Work out the finished part from the listing and answer in its coordinate system (mm). Face numbers are marked on the shaded views. A direction names the side the tool comes from. Round coordinates to 2 decimals unless told otherwise and drop trailing zeros. Order: outer loops, then holes, each group sorted by start corner. A loop starts at its lowest first (then second) coordinate and runs counter-clockwise, first axis right, second up. Notation, with made-up numbers: (72.5, 32) - (115.5, 32) arc R24 ccw to (115.5, 70) - close; hole circle Ø11 at (37.5, 80). An arc over 180 degrees is marked (long way). Put each result on its own line as item: value.
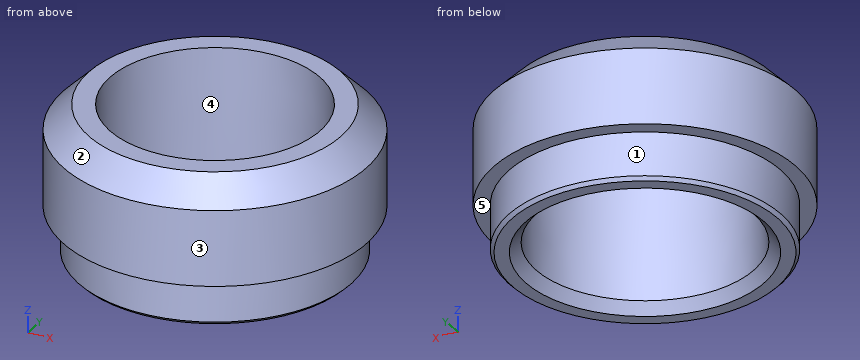
```python
from build123d import *

# Parameters (mm, degrees)
CHAMFER_SIZE    = 0.75
CHAMFER001_SIZE = 0.3
CHAMFER002_SIZE = 0.1


with BuildPart() as part:
    # Sketch → Revolution (revolve)
    with BuildSketch(Plane.XZ):
        Polygon((-4.5, 0), (-4.5, 3), (-3.125, 3), (-3.25, -1.4), (-4.05, -1.4), (-4.05, 0), align=None)
    revolve(axis=Axis((0, 0, 0), (0, 0, 1)))

    # Chamfer
    chamfer_edges = [part.edges().sort_by_distance(p)[0] for p in [
        (4.5, 0, 3),
    ]]
    chamfer(chamfer_edges, length=CHAMFER_SIZE)

    # Chamfer001
    chamfer001_edges = [part.edges().sort_by_distance(p)[0] for p in [
        (3.25, 0, -1.4),
    ]]
    chamfer(chamfer001_edges, length=CHAMFER001_SIZE)

    # Chamfer002
    chamfer002_edges = [part.edges().sort_by_distance(p)[0] for p in [
        (4.05, 0, -1.4),
    ]]
    chamfer(chamfer002_edges, length=CHAMFER002_SIZE)


solid = part.part
```
1) Given pin 1 Ø2 at (x, z) = (-3.5, 0) entering from +Y; pin 2 Ø2 at (x, z) = (3, -0.5) entering from +Y, each flat-ended and moving along its own axis, determine where each tip first touches the part or whether it passes through.
Findings below:
pin 1: stops at y = 3.74
pin 2: stops at y = 3.96
2) For a pull along X with two mould halves and no side action, classify the marked faces 3, 4 and 5 as pulls with the +X half, pulls with the -X half, needs draft (parallel to the pull), parting line crosses it, or undercut.
Findings below:
face 3: parting line crosses it
face 4: undercut
face 5: needs draft
3) Straight lines are drawn through the part: L1, parallel to Y at x = 1.25, z = 2; L2, parallel to X at y = 1, z = 1.3; L3, parallel to X at y = 0.25, z = 1.6. For each, find the intervals that lie inside material, in ascending order. Write a range as from..to.
Findings below:
L1: y = -4.32..-2.9, 2.9..4.32
L2: x = -4.39..-3.01, 3.01..4.39
L3: x = -4.49..-3.15, 3.15..4.49
4) A cutting plane is placed at A-A on x = 0. Write down the section's boundary in (y, z) (3 decimals).
Findings below:
outline: (-4.5, 0) - (-4.05, 0) - (-4.05, -1.3) - (-3.95, -1.4) - (-3.55, -1.4) - (-3.241, -1.1) - (-3.125, 3) - (-3.75, 3) - (-4.5, 2.25) - close; (3.125, 3) - (3.241, -1.1) - (3.55, -1.4) - (3.95, -1.4) - (4.05, -1.3) - (4.05, 0) - (4.5, 0) - (4.5, 2.25) - (3.75, 3) - close
5) A cutting plane is placed at C-C on z = 1.4. Write down the section's boundary in (x, y).
Findings below:
outline: circle Ø9 at (0, 0); hole circle Ø6.34 at (0, 0)
6) A cutting plane is placed at D-D on z = 0.65. Write down the section's boundary in (x, y).
Findings below:
outline: circle Ø9 at (0, 0); hole circle Ø6.38 at (0, 0)
7) For the marked faces 1 and 2, determine the directions among +Z, -Z, +X, -X, +Y, -Y from which every point of the face is accessible in a straight line to the end or side of a thin tool.
Findings below:
face 1: -Z
face 2: +Z
